CAD build for the part. Positions are in the model's coordinates, mm. Face numbers are marked on the shaded views. A direction names the side the tool comes from. Give positions to 0.01 mm unless a question says otherwise; leave off trailing zeros. Write each loop counter-clockwise with the first axis right and the second up, starting at its lowest first coordinate (ties: lowest second). Pieces come first, ordered by that corner, then holes. Notation, with made-up numbers: (-12, -38) -> (15, -38) arc R27 ccw to (15, -1) -> close; hole circle Ø7 at (1, -2.75). An arc over 180 degrees is marked (long way). Answer as a JSON object with one key per item and string values.
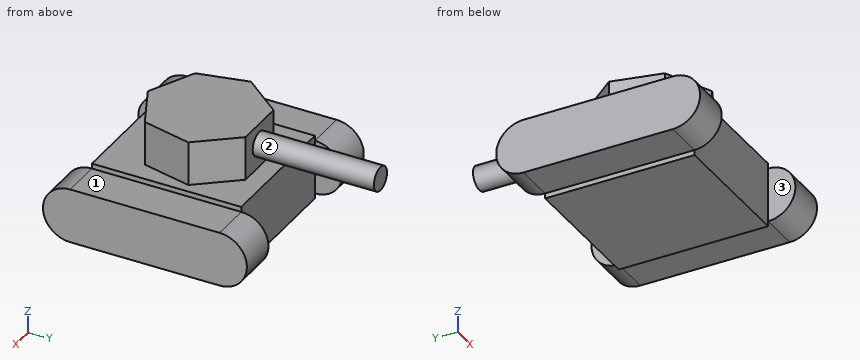
```python
from build123d import *

# Parameters (mm, degrees)
F0_W     = 52.6865217835
F0_H     = 58.567808941
F1_DEPTH = 25.4
F2_W     = 58.567808941
F2_H     = 21.3762959349
F3_DEPTH = 15.494
F7_DEPTH = 17.272
F8_R     = 4.6929987143
F9_DEPTH = 47.498


with BuildPart() as f1:
    # F0 (on Top) → F1 (new body)
    with BuildSketch(Plane.XY):
        with Locations((1.2252675369, -1.3477941975)):
            Rectangle(F0_W, F0_H)
    extrude(amount=F1_DEPTH)

    # F2 (on face) → F3 (join)
    with BuildSketch(Plane.YZ.offset(27.5685284287)):
        with BuildLine():
            Line((-30.631698668, 2.0118520325), (-30.631698668, 23.3881479675))
            ThreePointArc((-30.631698668, 23.3881479675), (-41.3198466355, 12.7), (-30.631698668, 2.0118520325))
        make_face()
        with Locations((-1.3477941975, 12.7)):
            Rectangle(F2_W, F2_H)
        with BuildLine():
            ThreePointArc((27.936110273, 2.0118520325), (38.6242582405, 12.7), (27.936110273, 23.3881479675))
            Line((27.936110273, 23.3881479675), (27.936110273, 2.0118520325))
        make_face()
    extrude(amount=F3_DEPTH)

    # F5: F1 across plane


with BuildPart() as f1_1:
    add(f1.part)
    add(f1.part.mirror(Plane(origin=(1.2252675369, -1.3477941975, 18.5470369919), x_dir=(0, 1, 0), z_dir=(1, 0, 0))))

    # F6 (on face) → F7 (join)
    with BuildSketch(Plane.XY.offset(25.4)):
        Polygon((11.3696932765, 20.753711462), (-8.6192280958, 20.753711462), (-21.0821167216, 5.1257434326), (-16.6341632691, -14.3620139477), (1.3752325904, -23.0348818937), (19.3846284498, -14.3620139477), (23.8325819023, 5.1257434326), align=None)
    extrude(amount=F7_DEPTH)

    # F8 (on face) → F9 (join)
    with BuildSketch(Plane(origin=(0, 20.753711462, 0), x_dir=(-1, 0, 0), z_dir=(0, 1, 0))):
        with Locations((-1.5616653254, 34.6986874938)):
            Circle(F8_R)
    extrude(amount=F9_DEPTH)


solid = f1_1.part
```
1) Slice it at A-A (z = 12.7). List the corners of the cut face in (x, y).
Model answer:
{"outline": "(-40.61, -41.32) -> (-25.12, -41.32) -> (-25.12, -30.63) -> (27.57, -30.63) -> (27.57, -41.32) -> (43.06, -41.32) -> (43.06, 38.62) -> (27.57, 38.62) -> (27.57, 27.94) -> (-25.12, 27.94) -> (-25.12, 38.62) -> (-40.61, 38.62) -> close"}
2) Slice it at D-D (x = -30.5). List the corners of the cut face in (y, z), then the cut area to 3 significant figures.
Model answer:
{"outline": "(-30.63, 2.01) -> (27.94, 2.01) arc R10.69 ccw to (27.94, 23.39) -> (-30.63, 23.39) arc R10.69 ccw to start", "area": "1,610 mm2"}
3) Slice it at C-C (y = -33). List the corners of the cut face in (x, z).
Model answer:
{"outline": "(-40.61, 2.28) -> (-25.12, 2.28) -> (-25.12, 23.12) -> (-40.61, 23.12) -> close; (27.57, 2.28) -> (43.06, 2.28) -> (43.06, 23.12) -> (27.57, 23.12) -> close"}
4) Slice it at B-B (y = 31.5). List the corners of the cut face in (x, z).
Model answer:
{"outline": "(-40.61, 2.62) -> (-25.12, 2.62) -> (-25.12, 22.78) -> (-40.61, 22.78) -> close; circle Ø9.39 at (1.56, 34.7); (27.57, 2.62) -> (43.06, 2.62) -> (43.06, 22.78) -> (27.57, 22.78) -> close"}
5) Wall check: probe 1 along Y at (x, z) = (-3.5, 16); probe 2 along Z at (x, y) = (38, 7); probe 3 along X at (y, z) = (-26.5, 25). Give the ranges that are in metal, low to high.
Model answer:
{"probe 1": "y = -30.63 to 27.94", "probe 2": "z = 2.01 to 23.39", "probe 3": "x = -25.12 to 27.57"}
6) 3-axis set-ups, long thin cutter, end or side, ignore diameter. For the marked faces 1, 2 and 3: which of +Z, -Z, +X, -X, +Y, -Y reach the whole face in a straight line?
Model answer:
{"face 1": "+Z, +X, +Y, -Y", "face 2": "+Y", "face 3": "+Z, -Z, -Y"}
7) Pin check, flat tips, straight feed: pin 1 (7.5 mm diameter, centred on x = 5, z = 18.5, fed in from -Y); pin 2 (4.5 mm diameter, centred on x = 38.5, y = -10.5, fed in from -Z); pin 3 (0.6 mm diameter, centred on y = 1.5, z = 24.5, fed in from -X). Stop position of each tip, or through.
Model answer:
{"pin 1": "stops at y = -30.63", "pin 2": "stops at z = 2.01", "pin 3": "stops at x = -25.12"}
